```python
from build123d import *

# Parameters (mm, degrees)
SKETCH1_W           = 119.144328959
SKETCH1_H           = 140.724589222
BOSS_EXTRUDE1_DEPTH = 10
SKETCH2_W           = 10
SKETCH2_H           = 20
SKETCH2_H_2         = 20.724589222
CUT_EXTRUDE1_DEPTH  = 10
CUT_EXTRUDE2_DEPTH  = 10
CUT_EXTRUDE6_DEPTH  = 150
CUT_EXTRUDE7_REACH  = 169.502
SKETCH9_W           = 10
SKETCH9_H           = 25.346761212
SKETCH10_W          = 31.040737262
SKETCH10_H          = 31.620202264
CUT_EXTRUDE8_DEPTH  = 150
FILLET1_R           = 10


with BuildPart() as part:
    # Sketch1 → Boss-Extrude1 (new body)
    with BuildSketch(Plane.XY):
        with Locations((59.57216448, 70.362294611)):
            Rectangle(SKETCH1_W, SKETCH1_H)
    extrude(amount=BOSS_EXTRUDE1_DEPTH)

    # Sketch2 → Cut-Extrude1 (cut)
    with BuildSketch(Plane.XY.offset(10)):
        with Locations((5, 50.724589222)):
            Rectangle(SKETCH2_W, SKETCH2_H)
        with Locations((5, 90.724589222)):
            Rectangle(SKETCH2_W, SKETCH2_H)
        with Locations((5, 10.362294611)):
            Rectangle(SKETCH2_W, SKETCH2_H_2)
        with Locations((5, 130.724589222)):
            Rectangle(SKETCH2_W, SKETCH2_H)
    extrude(amount=-CUT_EXTRUDE1_DEPTH, mode=Mode.SUBTRACT)

    # Sketch4 → Cut-Extrude2 (cut)
    with BuildSketch(Plane.XY.offset(10)):
        Polygon((10, 140.724589222), (119.144328959, 100.999302242), (119.144328959, 140.724589222), align=None)
    extrude(amount=-CUT_EXTRUDE2_DEPTH, mode=Mode.SUBTRACT)

    # Sketch7 → Cut-Extrude6 (cut)
    with BuildSketch(Plane.XY.offset(10)):
        Polygon((76.127978338, 92.605170498), (93.75776849, 110.239254603), (119.144328959, 100.999302242), (119.144328959, 0), (61.696670809, 0), (61.696670809, 78.170348045), align=None)
    extrude(amount=-CUT_EXTRUDE6_DEPTH, mode=Mode.SUBTRACT)

    # Cut-Extrude7: up to this plane
    cut_extrude7_end = Plane(origin=(241.768645896, -65.518758289, 505.407022073), z_dir=(0.6359690231741637, -0.635814162767, -0.4373599798653267))
    # Sketch9 → Cut-Extrude7 (cut, up to the surface)
    with BuildSketch(Plane(origin=(-8.22932488, 8.227321014, 0), x_dir=(0, 0, -1), z_dir=(0.7071928777614668, -0.7070206741273237, 0)), mode=Mode.PRIVATE) as cut_extrude7_sk1:
        with Locations((-5, 111.575715782)):
            Rectangle(SKETCH9_W, SKETCH9_H)
    cut_extrude7_tool1 = split(extrude(cut_extrude7_sk1.sketch, amount=-CUT_EXTRUDE7_REACH, mode=Mode.PRIVATE), bisect_by=cut_extrude7_end, keep=Keep.BOTH, mode=Mode.PRIVATE)
    add(cut_extrude7_tool1.solids().sort_by_distance((70.657013, 87.132873, 5))[0], mode=Mode.SUBTRACT)

    # Sketch10 → Cut-Extrude8 (cut)
    with BuildSketch(Plane(origin=(-9.939992949, 9.937572531, 6.835796961), x_dir=(-0.30929786277865773, 0.30922254780069597, -0.8992865216449099), z_dir=(0.6359690231741634, -0.6358141627670002, -0.4373599798653268))):
        with Locations((3.372258752, 133.362557089)):
            Rectangle(SKETCH10_W, SKETCH10_H)
    extrude(amount=CUT_EXTRUDE8_DEPTH, mode=Mode.SUBTRACT)

    # Fillet1
    fillet1_edges = [part.edges().sort_by_distance(p)[0] for p in [
        (90.324191509, 111.488974422, 5),
    ]]
    fillet(fillet1_edges, radius=FILLET1_R)


solid = part.part
```
Part model, mm, in its own coordinate system. A direction names the side the tool comes from. Round coordinates to 2 decimals unless told otherwise and drop trailing zeros. Loops run counter-clockwise (first coordinate to the right, second up) from the corner with the lowest first, then second, coordinate; pieces in that order, holes last.
Item 1: Cut at B-B, the plane x = 37.5. Give the cut face in (y, z).
Item 2: Drop flat-ended pins along their axis: P1, Ø3, axis at x = 6.5, z = 2.5, coming from the -Y side; P2, Ø5, axis at y = 50.5, z = 4.5, coming from the -X side; P3, Ø4, axis at x = 15, z = 2.5, coming from the +Y side. Give the stop position or say it passes through.
Item 3: Mould opens along Y. For faces 5 (the face through (78.521, 99.635, 5.07)), 6 (the face through (81.062, 110.264, 3.708)), 7 (the face through (5, 40.725, 5)) say: +Y half, -Y half, draft (parallel to the pull), parting line (faces both ways), or undercut.
Item 4: 3-axis set-ups, long thin cutter, end or side, ignore diameter. For faces 1 (the face through (5, 120.725, 5)), 2 (the face through (5, 60.725, 5)), 3 (the face through (5, 20.725, 5)), 4 (the face through (60.35, 97.19, 5.07)): which of +Z, -Z, +X, -X, +Y, -Y reach the whole face in a straight line?
Item 5: Drill centre lines: line 1 (Y direction, x = 8, z = 9); line 2 (X direction, y = 15, z = 0.75); line 3 (Y direction, x = 57, z = 8.25). Where is each one in solid material? Low to high.
Item 6: Cut at A-A, the plane y = 23. Give the cut face in (x, z), then the cut area to 3 significant figures.
A:
1. outline: (0, 0) - (130.72, 0) - (130.72, 10) - (0, 10) - close
2. P1: stops at y = 20.72
2. P2: stops at x = 10
2. P3: stops at y = 139.63
3. face 5: -Y half
3. face 6: parting line
3. face 7: undercut
4. face 1: +Z, -Z, -X, +Y
4. face 2: +Z, -Z, -X
4. face 3: +Z, -Z, -X, -Y
4. face 4: -Z
5. line 1: y = 20.72 to 40.72, 60.72 to 80.72, 100.72 to 120.72
5. line 2: x = 10 to 61.7
5. line 3: y = 0 to 82.87, 91.65 to 123.62
6. outline: (0, 0) - (61.7, 0) - (61.7, 10) - (0, 10) - close
6. area: 617 mm2
